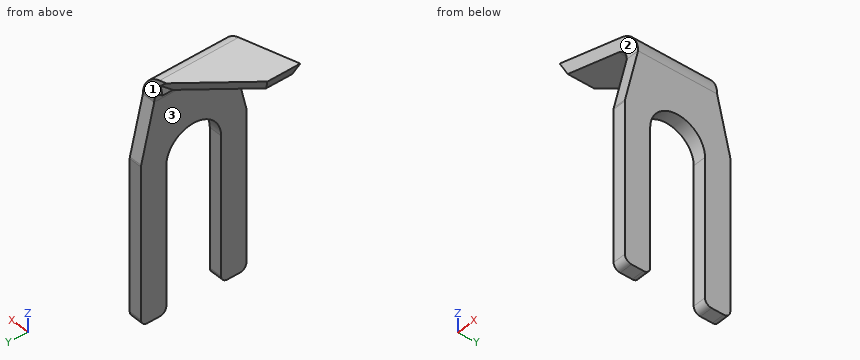
from build123d import *

# Parameters (mm, degrees)
BASE_FLANGE1_DEPTH  = 4.7625
CUT_EXTRUDE2_DEPTH  = 33.017769542
CUT_EXTRUDE3_REACH  = 35.526
TAB1_DEPTH          = 1.5875
BREAK_CORNER1_DEPTH = 1.5875
CUT_EXTRUDE7_REACH  = 32.474
SKETCH10_W          = 10.847778963
SKETCH10_H          = 1.122532015
CUT_EXTRUDE8_DEPTH  = 7.9375
CUT_EXTRUDE9_REACH  = 32.812
CUT_EXTRUDE4_DEPTH  = 35.511511322


# Read off the part's stored shape, not the designer's step: Break-Corner1
# Sheet-metal steps are written as plain solids
with BuildPart() as part:
    # Sketch1 → Base-Flange1 (new, symmetric)
    with BuildSketch(Plane(origin=(0, 0, 0), x_dir=(1, 0, 0), z_dir=(0, 1, 0))):
        with BuildLine():
            Line((0, 0), (0, -25.769368407))
            ThreePointArc((0, -25.769368407), (-0.328051572, -26.735777175), (-1.176624766, -27.302775656))
            Line((-1.176624766, -27.302775656), (-9.838340911, -29.623675502))
            Line((-9.838340911, -29.623675502), (-9.427465677, -31.157082751))
            Line((-9.427465677, -31.157082751), (-0.765749532, -28.836182905))
            ThreePointArc((-0.765749532, -28.836182905), (0.931396855, -27.702185944), (1.5875, -25.769368407))
            Line((1.5875, -25.769368407), (1.5875, 0))
            Line((1.5875, 0), (0, 0))
        make_face()
    extrude(amount=BASE_FLANGE1_DEPTH, both=True)

    # Sketch4 → Cut-Extrude2 (cut, through all)
    with BuildSketch(Plane(origin=(7.157750234, 0, 26.713087542), x_dir=(0.9659258262890691, 0, -0.2588190451025182), z_dir=(0.2588190451025182, 0, 0.9659258262890691))):
        Polygon((-17.17027898, 4.7625), (-17.17027898, -0.79375), (-9.162982379, 4.7625), align=None)
    extrude(amount=-CUT_EXTRUDE2_DEPTH, mode=Mode.SUBTRACT)

    # Sketch5 → Cut-Extrude3 (cut, up to next)
    with BuildSketch(Plane(origin=(1.5875, 0, 0), x_dir=(0, 0, -1), z_dir=(1, 0, 0)), mode=Mode.PRIVATE) as cut_extrude3_sk1:
        with BuildLine():
            Line((0, -3.302), (-17.4625, -3.302))
            ThreePointArc((-17.4625, -3.302), (-20.7645, 0), (-17.4625, 3.302))
            Line((-17.4625, 3.302), (0, 3.302))
            ThreePointArc((0, 3.302), (3.302, 0), (0, -3.302))
        make_face()
    cut_extrude3_tool1 = extrude(cut_extrude3_sk1.sketch, amount=-CUT_EXTRUDE3_REACH, mode=Mode.PRIVATE) & part.part
    add(cut_extrude3_tool1.solids().sort_by_distance((1.5875, 0, 8.73125))[0], mode=Mode.SUBTRACT)

    # Sketch6 → Tab1 (add)
    with BuildSketch(Plane(origin=(1.5875, 0, 0), x_dir=(0, 0, -1), z_dir=(1, 0, 0))):
        Polygon((-25.769368407, 4.7625), (0, 4.7625), (0, 6.35), (-19.05, 6.35), align=None)
        Polygon((0, -4.7625), (-25.769368407, -4.7625), (-19.05, -6.35), (0, -6.35), align=None)
    extrude(amount=-TAB1_DEPTH)

    # Break-Corner1 outline → Break-Corner1 (cut)
    with BuildSketch(Plane.YZ):
        with BuildLine():
            ThreePointArc((-3.302, 0.79375), (-3.534483992, 0.232483992), (-4.09575, 0))
            Line((-4.09575, 0), (-3.302, 0))
            Line((-3.302, 0), (-3.302, 0.79375))
        make_face()
        with BuildLine():
            ThreePointArc((-5.55625, 0), (-6.117516008, 0.232483992), (-6.35, 0.79375))
            Line((-6.35, 0.79375), (-6.35, 0))
            Line((-6.35, 0), (-5.55625, 0))
        make_face()
        with BuildLine():
            ThreePointArc((-6.35, 18.957508511), (-6.344665491, 19.049378398), (-6.328733667, 19.140013435))
            Line((-6.328733667, 19.140013435), (-6.35, 19.05))
            Line((-6.35, 19.05), (-6.35, 18.957508511))
        make_face()
        with BuildLine():
            Line((3.302, 0), (4.09575, 0))
            ThreePointArc((4.09575, 0), (3.534483992, 0.232483992), (3.302, 0.79375))
            Line((3.302, 0.79375), (3.302, 0))
        make_face()
        with BuildLine():
            Line((6.35, 0), (6.35, 0.79375))
            ThreePointArc((6.35, 0.79375), (6.117516008, 0.232483992), (5.55625, 0))
            Line((5.55625, 0), (6.35, 0))
        make_face()
        with BuildLine():
            ThreePointArc((6.328733667, 19.140013435), (6.344665491, 19.049378398), (6.35, 18.957508511))
            Line((6.35, 18.957508511), (6.35, 19.05))
            Line((6.35, 19.05), (6.328733667, 19.140013435))
        make_face()
    extrude(amount=BREAK_CORNER1_DEPTH, mode=Mode.SUBTRACT)

    # Cut-Extrude7: up to this plane
    cut_extrude7_end = Plane(origin=(0, 4.7625, 26.9875), z_dir=(0.25881904510251813, 0, 0.965925826289069))
    # Sketch10 → Cut-Extrude7 (cut, up to the surface)
    with BuildSketch(Plane(origin=(-5.368839639, 15.113767658, 20.483491715), x_dir=(0.7935854418944778, 0.5700930896630726, -0.21264057828071875), z_dir=(-0.20636811960864032, 0.5809448636137555, 0.7873469785615419)), mode=Mode.PRIVATE) as cut_extrude7_sk1:
        with Locations((-10.236945168, -12.533570263)):
            Rectangle(SKETCH10_W, SKETCH10_H)
    cut_extrude7_tool1 = split(extrude(cut_extrude7_sk1.sketch, amount=-CUT_EXTRUDE7_REACH, mode=Mode.PRIVATE), bisect_by=cut_extrude7_end, keep=Keep.BOTH, mode=Mode.PRIVATE)
    add(cut_extrude7_tool1.solids().sort_by_distance((-6.318596, 1.996443, 29.913188))[0], mode=Mode.SUBTRACT)

    # Sketch11 → Cut-Extrude8 (cut)
    with BuildSketch(Plane(origin=(7.495399471, -7.607377871, 7.577699232), x_dir=(0.819979057279916, 0.40553362238795987, -0.4039515153273222), z_dir=(-0.5723935233930764, 0.5809448636137574, -0.5786784252228975))):
        Polygon((-10.640638737, -21.79431173), (-10.575909421, -21.81114428), (-10.249235129, -23.422955447), (-10.344964483, -23.791081213), (-11.205664927, -23.967111285), align=None)
    extrude(amount=CUT_EXTRUDE8_DEPTH, mode=Mode.SUBTRACT)

    # Cut-Extrude9: up to this face of the body (flat: up to its plane)
    cut_extrude9_end = Plane(part.part.faces().sort_by_distance((-5.381060773, 1.282704756, 29.23921233))[0])
    # Sketch12 → Cut-Extrude9 (cut, up to the picked face)
    with BuildSketch(Plane(origin=(6.746875, 0, 25.179680292), x_dir=(-0.9659258262890691, 0, 0.25881904510251813), z_dir=(-0.25881904510251813, 0, -0.9659258262890691)), mode=Mode.PRIVATE) as cut_extrude9_sk1:
        Polygon((8.558950337, 4.7625), (8.203010573, 3.496370622), (8.203010573, 4.7625), align=None)
    cut_extrude9_tool1 = split(extrude(cut_extrude9_sk1.sketch, amount=-CUT_EXTRUDE9_REACH, mode=Mode.PRIVATE), bisect_by=cut_extrude9_end, keep=Keep.BOTH, mode=Mode.PRIVATE)
    add(cut_extrude9_tool1.solids().sort_by(Axis((-1.291229, 4.340457, 27.333484), (0.25881904510251813, 0, 0.9659258262890691)))[0], mode=Mode.SUBTRACT)

    # Sketch7 → Cut-Extrude4 (cut, through all)
    with BuildSketch(Plane.XZ.offset(4.7625)):
        Polygon((-9.427465677, 31.157082751), (-8.304933662, 29.212800268), (-9.838340911, 29.623675502), align=None)
    extrude(amount=-CUT_EXTRUDE4_DEPTH, mode=Mode.SUBTRACT)


solid = part.part
For this review, take the finished solid that the model builds, in its own axes (mm). Face numbers are marked on the shaded views. Round coordinates to 2 decimals unless told otherwise and drop trailing zeros. Loops run counter-clockwise (first coordinate to the right, second up) from the corner with the lowest first, then second, coordinate; pieces in that order, holes last. Notation, with made-up numbers: (-0.75, 44.5) - (27.25, 44.5) arc R20 cw to (27.25, 57.5) - close; hole circle Ø1 at (8, -8). An arc over 180 degrees is marked (long way). One line per question, with ' | ' between items.
Q1. Take a section at A-A (z = 6.5). Give the boundary of the cut face in (x, y), and give its area (3 significant figures).
Taken from the geometry:
outline: (0, -6.35) - (1.59, -6.35) - (1.59, -3.3) - (0, -3.3) - close; (0, 3.3) - (1.59, 3.3) - (1.59, 6.35) - (0, 6.35) - close | area: 9.68 mm²
Q2. Take a section at C-C (x = -7). Give the boundary of the cut face in (y, z), and give its area (3 significant figures).
Taken from the geometry:
outline: (-4.76, 28.86) - (-0.69, 28.86) - (0.95, 30.51) - (-4.76, 30.51) - close | area: 8.04 mm²
Q3. For line 1 along Y through (x, z) = (0.75, 12); line 2 along X through (y, z) = (-5, 8.5); line 3 along Z through (x, y) = (-6.75, -2.75), list the stretches that pass through material, from the lowest coordinate up. Write a range as [from, to].
Taken from the geometry:
line 1: y = [-6.35, -3.3], [3.3, 6.35] | line 2: x = [0, 1.59] | line 3: z = [28.8, 30.44]
Q4. For pin 1 (4 mm diameter, centred on x = -1.5, y = 1.5, fed in from -Z); pin 2 (1 mm diameter, centred on x = -1, z = 28, fed in from +Y); pin 3 (3 mm diameter, centred on x = -0.5, y = 4, fed in from +Z), all flat-tipped, find the tip position at first contact; note any pin that passes through.
Taken from the geometry:
pin 1: stops at z = 19.18 | pin 2: stops at y = 4.76 | pin 3: stops at z = 29.17
Q5. The part is to be moulded in two halves that separate along Y. For the marked faces 1, 2 and 3, say which applies: released by +Y, released by -Y, zero draft, split by the parting line, or undercut.
Taken from the geometry:
face 1: released by +Y | face 2: released by -Y | face 3: zero draft
